Design review of the part built by this model. Coordinates are the model's own, in mm. Face numbers are marked on the shaded views. Give positions to 0.01 mm unless a question says otherwise; leave off trailing zeros. Write each loop counter-clockwise with the first axis right and the second up, starting at its lowest first coordinate (ties: lowest second). Pieces come first, ordered by that corner, then holes. Notation, with made-up numbers: (83, -23) - (140, -23) arc R19 ccw to (140, -13) - close; hole circle Ø7 at (-37.75, -22). An arc over 180 degrees is marked (long way). Use a Markdown table: item, result. Add a question column.
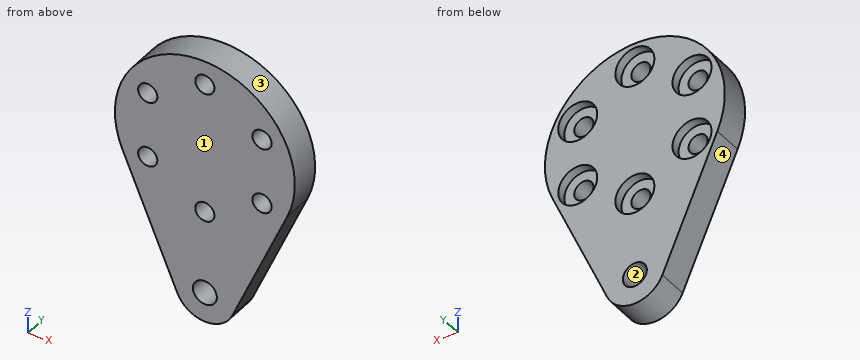
```python
from build123d import *

# Parameters (mm, degrees)
SKETCH4_R           = 2
SKETCH4_R_2         = 1.6
BOSS_EXTRUDE1_DEPTH = 5
SKETCH6_R           = 3.25
CUT_EXTRUDE1_DEPTH  = 1.5


with BuildPart() as part:
    # Sketch4 → Boss-Extrude1 (new body)
    with BuildSketch(Plane(origin=(0, 0, 0), x_dir=(1, 0, 0), z_dir=(0, 1, 0))):
        with BuildLine():
            Line((13.747727085, 6), (4.582575695, 27))
            ThreePointArc((4.582575695, 27), (0, 30), (-4.582575695, 27))
            Line((-4.582575695, 27), (-13.747727085, 6))
            ThreePointArc((-13.747727085, 6), (0, -15), (13.747727085, 6))
        make_face()
        with Locations((0, 25)):
            Circle(SKETCH4_R, mode=Mode.SUBTRACT)
        with Locations((0, 11)):
            Circle(SKETCH4_R_2, mode=Mode.SUBTRACT)
        with Locations((-9.526279442, -5.5)):
            Circle(SKETCH4_R_2, mode=Mode.SUBTRACT)
        with Locations((-9.526279442, 5.5)):
            Circle(SKETCH4_R_2, mode=Mode.SUBTRACT)
        with Locations((0, -11)):
            Circle(SKETCH4_R_2, mode=Mode.SUBTRACT)
        with Locations((9.526279442, -5.5)):
            Circle(SKETCH4_R_2, mode=Mode.SUBTRACT)
        with Locations((9.526279442, 5.5)):
            Circle(SKETCH4_R_2, mode=Mode.SUBTRACT)
    extrude(amount=BOSS_EXTRUDE1_DEPTH)

    # Sketch6 → Cut-Extrude1 (cut)
    with BuildSketch(Plane(origin=(0, 5, 0), x_dir=(1, 0, 0), z_dir=(0, 1, 0))):
        with Locations((0, 11)):
            Circle(SKETCH6_R)
        with Locations((9.526279442, 5.5)):
            Circle(SKETCH6_R)
        with Locations((9.526279442, -5.5)):
            Circle(SKETCH6_R)
        with Locations((0, -11)):
            Circle(SKETCH6_R)
        with Locations((-9.526279442, -5.5)):
            Circle(SKETCH6_R)
        with Locations((-9.526279442, 5.5)):
            Circle(SKETCH6_R)
    extrude(amount=-CUT_EXTRUDE1_DEPTH, mode=Mode.SUBTRACT)


solid = part.part
```
(1) Mouldability with a two-part tool opening along Z and no side actions: class the marked faces 1, 2, 3 and 4 as +Z half, -Z half, draft (parallel to the pull), parting line (faces both ways), or undercut.
(2) Add section B-B (z = -24.5). State the section outline as (x, y) points.
(3) Insertion check: pin 1 (2.5 mm diameter, centred on x = 9.53, z = 5.5, fed in from +Y); pin 2 (3 mm diameter, centred on x = -11, z = 6, fed in from +Y); pin 3 (1 mm diameter, centred on y = 2, z = -7, fed in from -X); pin 4 (2 mm diameter, centred on y = 3.5, z = -16, fed in from -X). Each pin has a flat end and moves straight along its axis. Give the tip position at first contact, or say it passes through.
(4) Add section A-A (x = 0). State the section outline as (y, z) points.
(5) Add section C-C (y = 0.5). State the section outline as (x, z) points, and give its area (3 significant figures).
(6) Add section D-D (x = 9). State the section outline as (y, z) points, and give its area (3 significant figures).
(7) For line 1 along Z through (x, y) = (0, 4.5); line 2 along Z through (x, y) = (0, 0.8); line 3 along Z through (x, y) = (-12.5, 3.65), list the stretches that pass through material, from the lowest coordinate up.
Answers follow:
| question | item | result |
|---|---|---|
| 1 | face 1 | draft |
| 1 | face 2 | undercut |
| 1 | face 3 | parting line |
| 1 | face 4 | -Z half |
| 2 | outline | (-5.67, 0) - (-1.94, 0) - (-1.94, 5) - (-5.67, 5) - close; (1.94, 0) - (5.67, 0) - (5.67, 5) - (1.94, 5) - close |
| 3 | pin 1 | through |
| 3 | pin 2 | y = 3.5 |
| 3 | pin 3 | x = -13.53 |
| 3 | pin 4 | x = -9.82 |
| 4 | outline | (0, -30) - (5, -30) - (5, -27) - (0, -27) - close; (0, -23) - (5, -23) - (5, -14.25) - (3.5, -14.25) - (3.5, -12.6) - (0, -12.6) - close; (0, -9.4) - (3.5, -9.4) - (3.5, -7.75) - (5, -7.75) - (5, 7.75) - (3.5, 7.75) - (3.5, 9.4) - (0, 9.4) - close; (0, 12.6) - (3.5, 12.6) - (3.5, 14.25) - (5, 14.25) - (5, 15) - (0, 15) - close |
| 5 | outline | (-13.75, -6) - (-4.58, -27) arc R5 ccw to (4.58, -27) - (13.75, -6) arc R15 ccw (long way) to start; hole circle Ø3.2 at (-9.53, -5.5); hole circle Ø3.2 at (-9.53, 5.5); hole circle Ø4 at (0, -25); hole circle Ø3.2 at (0, -11); hole circle Ø3.2 at (0, 11); hole circle Ø3.2 at (9.53, -5.5); hole circle Ø3.2 at (9.53, 5.5) |
| 5 | area | 872 mm^2 |
| 6 | outline | (0, -16.88) - (5, -16.88) - (5, -8.71) - (3.5, -8.71) - (3.5, -7.01) - (0, -7.01) - close; (0, -3.99) - (3.5, -3.99) - (3.5, -2.29) - (5, -2.29) - (5, 2.29) - (3.5, 2.29) - (3.5, 3.99) - (0, 3.99) - close; (0, 7.01) - (3.5, 7.01) - (3.5, 8.71) - (5, 8.71) - (5, 12) - (0, 12) - close |
| 6 | area | 104 mm^2 |
| 7 | line 1 | -30 to -27, -23 to -14.25, -7.75 to 7.75, 14.25 to 15 |
| 7 | line 2 | -30 to -27, -23 to -12.6, -9.4 to 9.4, 12.6 to 15 |
| 7 | line 3 | -8.86 to -6.81, -4.19 to 4.19, 6.81 to 8.29 |
